```python
from build123d import *

# Parameters (mm, degrees)
Y_KSEKLIK_EKSTR_ZYON2_DEPTH = 499.5
IZIM4_R                     = 2.5
Y_KSEKLIK_EKSTR_ZYON3_DEPTH = 5
IZIM5_R                     = 2.5
Y_KSEKLIK_EKSTR_ZYON4_DEPTH = 5


with BuildPart() as part:
    # Çizim2 → Yükseklik-Ekstrüzyon2 (new body)
    with BuildSketch(Plane(origin=(0, 0, 0), x_dir=(0, 0, -1), z_dir=(1, 0, 0))):
        Polygon((-25, 0), (25, 0), (25, 7.96), align=None)
    extrude(amount=Y_KSEKLIK_EKSTR_ZYON2_DEPTH)

    # Çizim4 → Yükseklik-Ekstrüzyon3 (add)
    with BuildSketch(Plane(origin=(499.5, 0, 0), x_dir=(0, 0, -1), z_dir=(1, 0, 0))):
        with Locations((20, 3.98)):
            Circle(IZIM4_R)
    extrude(amount=Y_KSEKLIK_EKSTR_ZYON3_DEPTH)

    # Çizim5 → Yükseklik-Ekstrüzyon4 (add)
    with BuildSketch(Plane.ZY):
        with Locations((-20, 3.98)):
            Circle(IZIM5_R)
    extrude(amount=Y_KSEKLIK_EKSTR_ZYON4_DEPTH)


solid = part.part
```
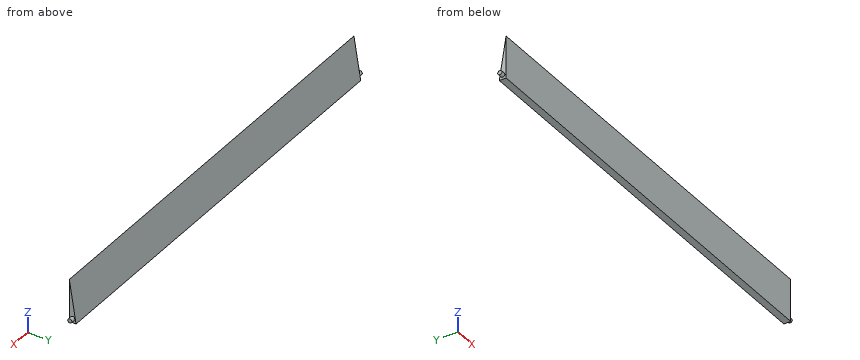
The model under review builds one solid part; all positions refer to its coordinate system, in mm. Round coordinates to 2 decimals unless told otherwise and drop trailing zeros. Order: outer loops, then holes, each group sorted by start corner. A loop starts at its lowest first (then second) coordinate and runs counter-clockwise, first axis right, second up. Notation, with made-up numbers: (20, -1) -> (68, -1) arc R26 ccw to (68, 18) -> close; hole circle Ø11 at (71, -23). An arc over 180 degrees is marked (long way). One line per item, written item: value. Start each with the question number.
Q1. Take a section at B-B (x = 382). Write out the cut boundary in (y, z).
Q2. Clearance check with flat-ended pins moving along their axes: pin 1 Ø3 at (y, z) = (3, 14) entering from -X; pin 2 Ø12 at (x, z) = (141.5, -5) entering from +Y; pin 3 Ø1 at (x, z) = (444.5, -3.5) entering from +Y. State where each tip first meets the part, or that it passes through.
Q3. Take a section at A-A (y = 3.98). Write out the cut boundary in (x, z), and give its area (3 significant figures).
Q4. Take a section at C-C (z = 19). Write out the cut boundary in (x, y).
Q5. Wall thickness on line 1 (X direction, y = 1.5, z = 7); line 2 (Y direction, x = 179, z = -6.5); line 3 (Y direction, x = 121.5, z = 20.5): over which ranges is each line inside the solid? List them lowest first.
Q6. Take a section at D-D (z = -8.5). Write out the cut boundary in (x, y), and give its area (3 significant figures).
Reported:
1. outline: (0, -25) -> (7.96, -25) -> (0, 25) -> close
2. pin 1: stops at x = 0
2. pin 2: stops at y = 5.73
2. pin 3: stops at y = 4.62
3. outline: (-5, -22.5) -> (0, -22.5) -> (0, -25) -> (499.5, -25) -> (499.5, -22.5) -> (504.5, -22.5) -> (504.5, -17.5) -> (499.5, -17.5) -> (499.5, 0) -> (0, 0) -> (0, -17.5) -> (-5, -17.5) -> close
3. area: 12,500 mm2
4. outline: (0, 0) -> (499.5, 0) -> (499.5, 0.96) -> (0, 0.96) -> close
5. line 1: x = 0 to 499.5
5. line 2: y = 0 to 5.01
5. line 3: y = 0 to 0.72
6. outline: (0, 0) -> (499.5, 0) -> (499.5, 5.33) -> (0, 5.33) -> close
6. area: 2,660 mm2
